Design review of the part built by this model. Coordinates are the model's own, in mm. Give positions to 0.01 mm unless a question says otherwise; leave off trailing zeros. Loops run counter-clockwise (first coordinate to the right, second up) from the corner with the lowest first, then second, coordinate; pieces in that order, holes last. Notation, with made-up numbers: M 29.25,31.25 L 81.25,31.25 A11 cw 81.25,47.25 Z; hole C 12,30 d10. An arc over 180 degrees is marked long. Answer as CSV lines item,"result".
```python
from build123d import *

# Parameters (mm, degrees)
F0_W     = 244
F0_H     = 122
F1_DEPTH = 10
F2_ANGLE = 90
F3_ANGLE = 125


with BuildPart() as f1:
    # F0 (on Top) → F1 (new body)
    with BuildSketch(Plane.XY):
        with Locations((0.335931778, -17.06091269)):
            Rectangle(F0_W, F0_H)
    extrude(amount=F1_DEPTH)


with BuildPart() as f1_1:
    # F2: moved
    add(f1.part.rotate(Axis((0.335931778, -78.06091269, 0), (1, 0, 0)), F2_ANGLE))


with BuildPart() as f1_2:
    # F3: moved
    add(f1_1.part.rotate(Axis((-121.664068222, -88.06091269, 61), (0, 0, -1)), F3_ANGLE))


solid = f1_2.part
```
1. To check wall thickness, follow L1, parallel to Y at x = -202, z = 68.5; L2, parallel to Y at x = -249, z = 48.5; L3, parallel to X at y = -236, z = 45. State the ranges of each line that lie inside material, in increasing order. Write a range as [from, to].
Answer block:
L1,"[-220.23, -202.79]"
L2,"[-287.35, -269.92]"
L3,"[-225.25, -213.04]"
2. We need section B-B, the plane x = -180. Write out the cut boundary in (y, z), plus the area to 3 significant figures.
Answer block:
outline,"M -188.81,0 L -171.37,0 L -171.37,122 L -188.81,122 Z"
area,"2,130 mm²"
3. We need section A-A, the plane z = 29.5. Write out the cut boundary in (x, y), plus the area to 3 significant figures.
Answer block:
outline,"M -261.62,-287.93 L -253.43,-293.67 L -113.47,-93.8 L -121.66,-88.06 Z"
area,"2,440 mm²"
4. For P1, Ø12, axis at y = -260, z = 106.5, coming from the +X side; P2, Ø3, axis at x = -211.5, z = 69.5, coming from the +Y side; P3, Ø2, axis at x = -200.5, y = -215, coming from the -Z side; P4, Ø3, axis at y = -252.5, z = 75, coming from the +X side, all flat-tipped, find the tip position at first contact; note any pin that passes through.
Answer block:
P1,"x = -225.65"
P2,"y = -214.22"
P3,"z = 0"
P4,"x = -223.55"
